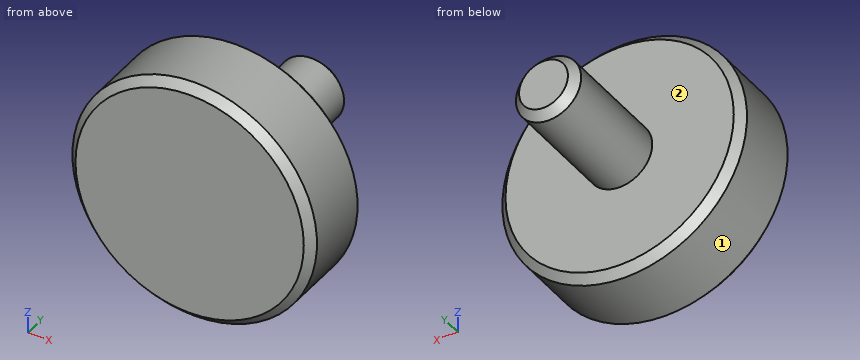
from build123d import *

# Parameters (mm, degrees)
CHAMFER_1_SIZE = 1


with BuildPart() as part:
    # Эскиз1 → Повернуть1 (revolve)
    with BuildSketch(Plane.XY, mode=Mode.PRIVATE) as revolve_1_sk:
        Polygon((0, 25), (4, 25), (4, 10), (15, 10), (15, 0), (0, 0), align=None)
    revolve(revolve_1_sk.sketch.rotate(Axis((0, 0, 0), (0, 1, 0)), 90), axis=Axis((0, 0, 0), (0, 1, 0)))

    # Фаска1
    chamfer_1_edges = [part.edges().sort_by_distance(p)[0] for p in [
        (0, 0, 15),
        (0, 10, 15),
        (0, 25, 4),
    ]]
    chamfer(chamfer_1_edges, length=CHAMFER_1_SIZE)


solid = part.part
Read the model definition and answer for the solid it produces. Units are mm, in the model's axes. Face numbers are marked on the shaded views. A direction names the side the tool comes from. Coordinates: 2 decimals unless noted, no trailing zeros. Loops run counter-clockwise (first coordinate to the right, second up) from the corner with the lowest first, then second, coordinate; pieces in that order, holes last. Notation, with made-up numbers: (-21, -1.5) -> (-15, -1.5) arc R38 cw to (-15, 36.5) -> close; hole circle Ø2 at (87.5, 62.5). An arc over 180 degrees is marked (long way). Answer in a Markdown table with one row per item.
Item 1: Straight lines are drawn through the part: line 1 along Y through (x, z) = (-5.25, 2); line 2 along X through (y, z) = (8.5, -12.25); line 3 along X through (y, z) = (7.5, -5.75). For each, find the intervals that lie inside material, in ascending order. Write a range as [from, to].
Returned:
| item | result |
|---|---|
| line 1 | y = [0, 10] |
| line 2 | x = [-8.66, 8.66] |
| line 3 | x = [-13.85, 13.85] |
Item 2: A cutting plane is placed at D-D on y = 2.25. Determine the outline of the cut face in (x, z).
Returned:
| item | result |
|---|---|
| outline | circle Ø30 at (0, 0) |
Item 3: A cutting plane is placed at A-A on z = 0. Determine the outline of the cut face in (x, y).
Returned:
| item | result |
|---|---|
| outline | (-15, 1) -> (-14, 0) -> (14, 0) -> (15, 1) -> (15, 9) -> (14, 10) -> (4, 10) -> (4, 24) -> (3, 25) -> (-3, 25) -> (-4, 24) -> (-4, 10) -> (-14, 10) -> (-15, 9) -> close |
Item 4: A cutting plane is placed at C-C on y = 19.75. Determine the outline of the cut face in (x, z).
Returned:
| item | result |
|---|---|
| outline | circle Ø8 at (0, 0) |
Item 5: Each of these flat-tipped pins is pushed along its axis until it touches: P1, Ø6, axis at x = -6, z = -8, coming from the +Y side; P2, Ø6, axis at y = 4.5, z = 4.5, coming from the -X side; P3, Ø5, axis at y = 13, z = -9, coming from the +X side; P4, Ø5, axis at x = -8.5, y = 3, coming from the +Z side. Where does it stop, or does it pass through?
Returned:
| item | result |
|---|---|
| P1 | stops at y = 10 |
| P2 | stops at x = -14.92 |
| P3 | passes through |
| P4 | stops at z = 13.75 |
Item 6: For the marked faces 1 and 2, determine the directions among +Z, -Z, +X, -X, +Y, -Y from which every point of the face is accessible in a straight line to the end or side of a thin tool.
Returned:
| item | result |
|---|---|
| face 1 | +Y, -Y |
| face 2 | +Y |
Item 7: A cutting plane is placed at B-B on x = 0. Determine the outline of the cut face in (y, z), plus the area to 3 significant figures.
Returned:
| item | result |
|---|---|
| outline | (0, -14) -> (1, -15) -> (9, -15) -> (10, -14) -> (10, -4) -> (24, -4) -> (25, -3) -> (25, 3) -> (24, 4) -> (10, 4) -> (10, 14) -> (9, 15) -> (1, 15) -> (0, 14) -> close |
| area | 417 mm^2 |
